from build123d import *

# Parameters (mm, degrees)
SKETCH1_R               = 33
BOSS_EXTRUDE1_DEPTH     = 313.5
SKETCH2_R               = 31.34
BOSS_EXTRUDE2_DEPTH     = 200
CUT_EXTRUDE1_DEPTH      = 6
CUT_EXTRUDE2_DEPTH      = 516.616378729
CUT_EXTRUDE2_DEPTH_BACK = 516.616378729
SKETCH5_R               = 11


with BuildPart() as part:
    # Sketch1 → Boss-Extrude1 (new body)
    with BuildSketch(Plane(origin=(0, 0, 0), x_dir=(1, 0, 0), z_dir=(0, 1, 0))):
        with Locations(Location((0, 0, 0), (0, 0, 270))):
            Circle(SKETCH1_R)
    extrude(amount=BOSS_EXTRUDE1_DEPTH)

    # Sketch2 → Boss-Extrude2 (add)
    with BuildSketch(Plane(origin=(0, 313.5, 0), x_dir=(1, 0, 0), z_dir=(0, 1, 0))):
        with Locations(Location((0, 0, 0), (0, 0, 270))):
            Circle(SKETCH2_R)
    extrude(amount=BOSS_EXTRUDE2_DEPTH)

    # Sketch3 → Cut-Extrude1 (cut)
    with BuildSketch(Plane(origin=(33, 0, 0), x_dir=(0, 0, -1), z_dir=(1, 0, 0))):
        with BuildLine():
            Line((-10, 119), (-10, 0))
            Line((-10, 0), (10, 0))
            Line((10, 0), (10, 119))
            ThreePointArc((10, 119), (0, 129), (-10, 119))
        make_face()
    extrude(amount=-CUT_EXTRUDE1_DEPTH, mode=Mode.SUBTRACT)

    # Sketch5 → Cut-Extrude2 (cut, two sides: drawn at the far end of the back side and taken through both)
    with BuildSketch(Plane(origin=(0, 0, 0), x_dir=(0, 0, -1), z_dir=(1, 0, 0)).offset(-CUT_EXTRUDE2_DEPTH_BACK)):
        with Locations((0, 463.5)):
            Circle(SKETCH5_R)
        with Locations((0, 363.5)):
            Circle(SKETCH5_R)
    extrude(amount=CUT_EXTRUDE2_DEPTH + CUT_EXTRUDE2_DEPTH_BACK, mode=Mode.SUBTRACT)


solid = part.part
Geometry: final body of the model. Coordinates: model frame, mm. A direction names the side the tool comes from. Coordinates: 2 decimals unless noted, no trailing zeros. Order: outer loops, then holes, each group sorted by start corner. A loop starts at its lowest first (then second) coordinate and runs counter-clockwise, first axis right, second up.
(1) Section query A-A (z = -1.5). Return the cut outline in (x, y), plus the area to 3 significant figures.
(2) Draft query along Z for faces 1 (the face through (-32.215, 154.556, -7.154)), 2 (the face through (-12.1, 313.5, 29.2)), 3 (the face through (29, 129, 0)), 4 (the face through (-0.44, 452.76, 2.38)). Return one class per face: pulls with the +Z half, pulls with the -Z half, needs draft (parallel to the pull), parting line crosses it, or undercut.
(3) Section query C-C (y = 320). Return the cut outline in (x, z).
(4) Access query for faces 5 (the face through (27, 65, 0)), 6 (the face through (0, 513.5, 0)), 7 (the face through (-12, 412.1, 28.95)). Directions: +Z, -Z, +X, -X, +Y, -Y. A direction counts if a zero-diameter tool reaches every point of the face in a straight line with its end or side. Return the directions, or none.
(5) First-contact query: pin 1 (22 mm diameter, centred on y = 80.5, z = -1.5, fed in from +X); pin 2 (2 mm diameter, centred on y = 194.5, z = -12.5, fed in from -X); pin 3 (1 mm diameter, centred on x = -12.5, y = 272.5, fed in from +Z). Flat tips, straight axial feed; report the tip coordinate or a pass-through.
(6) Material intervals for probe 1 along Y at (x, z) = (15, 0); probe 2 along X at (y, z) = (104.5, 1); probe 3 along Z at (x, y) = (0.5, 463.5), sorted ascending.
(7) Section query D-D (z = -24). Return the cut outline in (x, y).
(8) Section query B-B (x = 0). Return the cut outline in (y, z), plus the area to 3 significant figures.
Solution:
1. outline: (-32.97, 0) - (27, 0) - (27, 128.89) - (32.97, 128.89) - (32.97, 313.5) - (31.3, 313.5) - (31.3, 352.6) - (-31.3, 352.6) - (-31.3, 313.5) - (-32.97, 313.5) - close; (-31.3, 374.4) - (31.3, 374.4) - (31.3, 452.6) - (-31.3, 452.6) - close; (-31.3, 474.4) - (31.3, 474.4) - (31.3, 513.5) - (-31.3, 513.5) - close
1. area: 29,700 mm2
2. face 1: parting line crosses it
2. face 2: needs draft
2. face 3: undercut
2. face 4: undercut
3. outline: circle Ø62.68 at (0, 0)
4. face 5: +X, -Y
4. face 6: +Z, -Z, +X, -X, +Y
4. face 7: +Y
5. pin 1: stops at x = 31.45
5. pin 2: stops at x = -30.93
5. pin 3: stops at z = 30.74
6. probe 1: y = 0 to 352.5, 374.5 to 452.5, 474.5 to 513.5
6. probe 2: x = -32.98 to 27
6. probe 3: z = -31.34 to -11, 11 to 31.34
7. outline: (-22.65, 0) - (22.65, 0) - (22.65, 313.5) - (20.15, 313.5) - (20.15, 513.5) - (-20.15, 513.5) - (-20.15, 313.5) - (-22.65, 313.5) - close
8. outline: (0, -33) - (313.5, -33) - (313.5, -31.34) - (513.5, -31.34) - (513.5, 31.34) - (313.5, 31.34) - (313.5, 33) - (0, 33) - close; hole circle Ø22 at (363.5, 0); hole circle Ø22 at (463.5, 0)
8. area: 32,500 mm2
